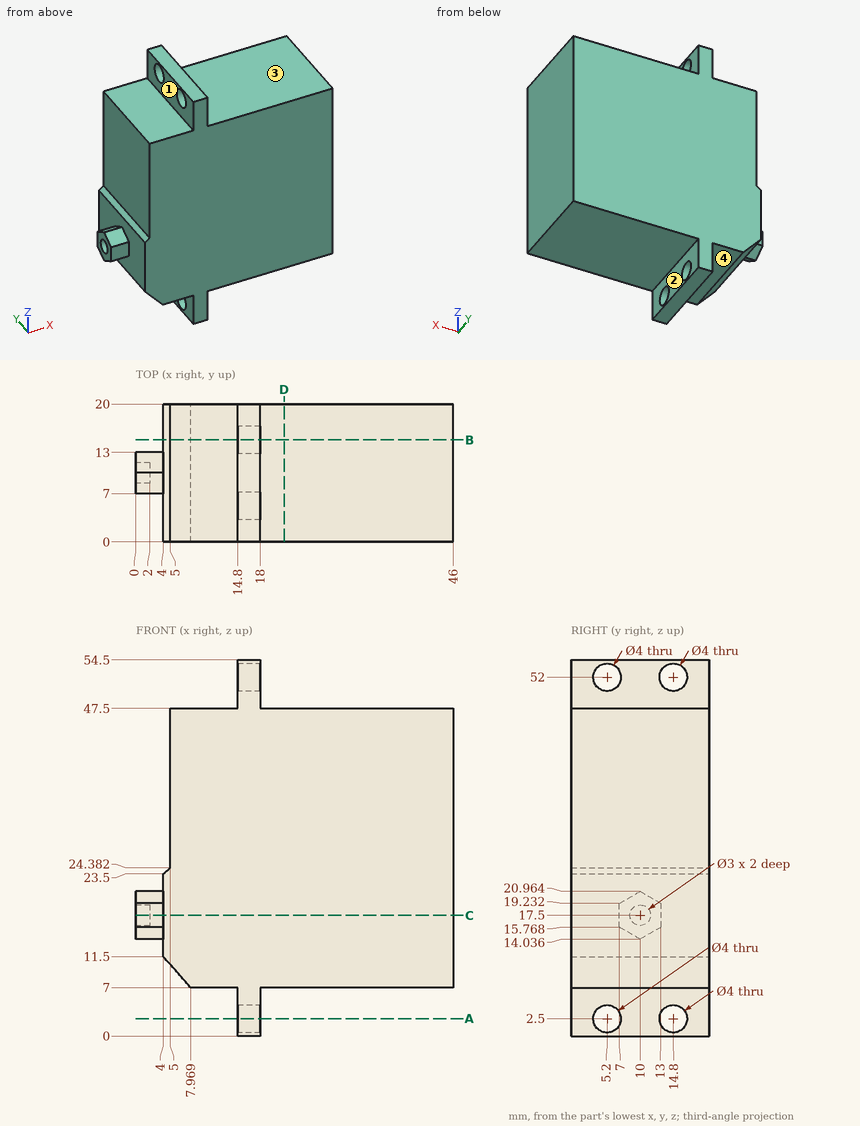
Could you check a few things on this drawing? It's one solid part, dimensions in mm from its lowest x, y, z. A direction names the side the tool comes from. Give positions to 0.01 mm unless a question says otherwise; leave off trailing zeros. Order: outer loops, then holes, each group sorted by start corner. A loop starts at its lowest first (then second) coordinate and runs counter-clockwise, first axis right, second up. Notation, with made-up numbers: (-27.5, 72.25) - (-22.5, 72.25) arc R8 cw to (-22.5, 87.25) - close; hole circle Ø8 at (19, 62). An arc over 180 degrees is marked (long way). Answer as a JSON object with one key per item and string values. Group by question number.
Item 1: If we section it at D-D on x = 21.5: Please give me the cut outline in (y, z), and give its area (3 significant figures).
Item 2: Which directions (+Z, -Z, +X, -X, +Y, -Y) give clear straight access to the entire face, cutting with the end or side of a thin tool? Please do the marked faces 1, 2, 3 and 4.
Item 3: Please list where these lines run through material, in increasing order: probe 1 along Y at (x, z) = (16.45, 52); probe 2 along Y at (x, z) = (17.5, 51); probe 3 along X at (y, z) = (18, 42).
Item 4: If we section it at A-A on z = 2.5: Please give me the cut outline in (x, y), and give its area (3 significant figures).
Item 5: If we section it at B-B on y = 14.8: Please give me the cut outline in (x, z), and give its area (3 significant figures).
Item 6: If we section it at C-C on z = 17.5: Please give me the cut outline in (x, y), and give its area (3 significant figures).
Item 7: For P1, Ø5, axis at y = 5.2, z = 2.5, coming from the -X side; P2, Ø3, axis at y = 15, z = 30, coming from the -X side; P3, Ø6, axis at x = 29.5, y = 11.5, coming from the -Z side; P4, Ø4, axis at x = 15, z = 33, coming from the -Y side, each with a flat end and sliding along its axis, tell me the tip position at first contact or that it passes through.
Result set:
{
 "1": {"outline": "(0, 7) - (20, 7) - (20, 47.5) - (0, 47.5) - close", "area": "810 mm²"},
 "2": {"face 1": "+Z, -X, +Y, -Y", "face 2": "-Z, +X, +Y, -Y", "face 3": "+Z, +X, +Y, -Y", "face 4": "-Z, -X, +Y, -Y"},
 "3": {"probe 1": "0 to 3.2, 7.2 to 12.8, 16.8 to 20", "probe 2": "0 to 3.47, 6.93 to 13.07, 16.53 to 20", "probe 3": "5 to 46"},
 "4": {"outline": "(14.8, 0) - (18, 0) - (18, 3.2) - (14.8, 3.2) - close; (14.8, 7.2) - (18, 7.2) - (18, 12.8) - (14.8, 12.8) - close; (14.8, 16.8) - (18, 16.8) - (18, 20) - (14.8, 20) - close", "area": "38.4 mm²"},
 "5": {"outline": "(4, 11.5) - (7.97, 7) - (14.8, 7) - (14.8, 4.5) - (18, 4.5) - (18, 7) - (46, 7) - (46, 47.5) - (18, 47.5) - (18, 50) - (14.8, 50) - (14.8, 47.5) - (5, 47.5) - (5, 24.38) - (4, 23.5) - close; (14.8, 0) - (18, 0) - (18, 0.5) - (14.8, 0.5) - close; (14.8, 54) - (18, 54) - (18, 54.5) - (14.8, 54.5) - close", "area": "1,690 mm²"},
 "6": {"outline": "(0, 7) - (4, 7) - (4, 0) - (46, 0) - (46, 20) - (4, 20) - (4, 13) - (0, 13) - (0, 11.5) - (2, 11.5) - (2, 8.5) - (0, 8.5) - close", "area": "858 mm²"},
 "7": {"P1": "x = 14.8", "P2": "x = 5", "P3": "z = 7", "P4": "y = 0"}
}
